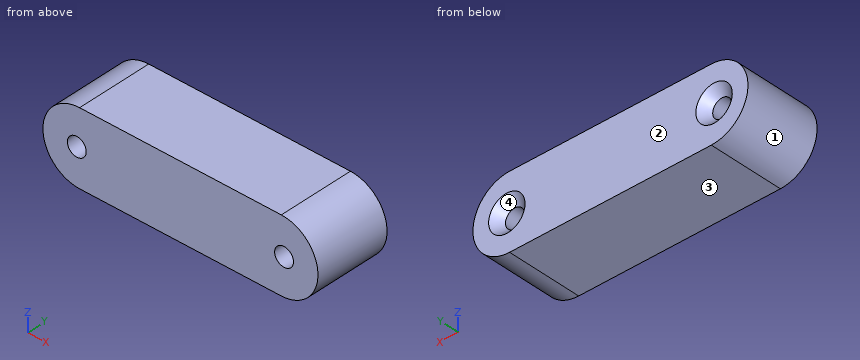
```python
from build123d import *

# Parameters (mm, degrees)
SKETCH1_R           = 1.905
BOSS_EXTRUDE1_DEPTH = 15.24
CHAMFER1_SIZE       = 1.778


with BuildPart() as part:
    # Sketch1 → Boss-Extrude1 (new body)
    with BuildSketch(Plane(origin=(0, 0, 0), x_dir=(1, 0, 0), z_dir=(0, 1, 0))):
        with BuildLine():
            Line((-20.3962, 7.4168), (20.3962, 7.4168))
            ThreePointArc((20.3962, 7.4168), (27.813, 0), (20.3962, -7.4168))
            Line((20.3962, -7.4168), (-20.3962, -7.4168))
            ThreePointArc((-20.3962, -7.4168), (-27.813, 0), (-20.3962, 7.4168))
        make_face()
        with Locations(Location((-20.955, 0, 0), (0, 0, 90))):
            Circle(SKETCH1_R, mode=Mode.SUBTRACT)
        with Locations(Location((20.955, 0, 0), (0, 0, 90))):
            Circle(SKETCH1_R, mode=Mode.SUBTRACT)
    extrude(amount=BOSS_EXTRUDE1_DEPTH)

    # Chamfer1
    chamfer1_edges = [part.edges().sort_by_distance(p)[0] for p in [
        (-20.955, 15.24, 1.905),
        (20.955, 15.24, 1.905),
    ]]
    chamfer(chamfer1_edges, length=CHAMFER1_SIZE)


solid = part.part
```
The model under review builds one solid part; all positions refer to its coordinate system, in mm. Face numbers are marked on the shaded views. Round coordinates to 2 decimals unless told otherwise and drop trailing zeros. Loops run counter-clockwise (first coordinate to the right, second up) from the corner with the lowest first, then second, coordinate; pieces in that order, holes last. Notation, with made-up numbers: (-24, 72.25) - (-17, 72.25) arc R19 cw to (-17, 96.25) - close; hole circle Ø3 at (-27, -35.75). An arc over 180 degrees is marked (long way). Use a Markdown table: item, result. Add a question column.
Q1. Add section A-A (z = 0). State the section outline as (x, y) points.
Q2. Add section C-C (z = -5.5). State the section outline as (x, y) points.
Q3. The part is to be moulded in two halves that separate along Z. For the marked faces 1, 2, 3 and 4, say which applies: pulls with the +Z half, pulls with the -Z half, needs draft (parallel to the pull), parting line crosses it, or undercut.
Q4. Insertion check: pin 1 Ø6 at (x, z) = (-20.955, 0) entering from +Y; pin 2 Ø3 at (y, z) = (11, 5) entering from +X; pin 3 Ø2 at (y, z) = (12.5, 5) entering from -X. Each pin has a flat end and moves straight along its axis. Give the tip position at first contact, or say it passes through.
Q5. For probe 1 along X at (y, z) = (8.25, 0); probe 2 along X at (y, z) = (3.75, -0.5); probe 3 along Z at (x, y) = (23, 14.5), list the stretches that pass through material, from the lowest coordinate up.
Q6. Add section B-B (y = 2). State the section outline as (x, z) points (3 decimals), plus the area to 3 significant figures.
Worked answers:
| question | item | result |
|---|---|---|
| 1 | outline | (-27.81, 0) - (-22.86, 0) - (-22.86, 13.46) - (-24.64, 15.24) - (-27.81, 15.24) - close; (-19.05, 0) - (19.05, 0) - (19.05, 13.46) - (17.27, 15.24) - (-17.27, 15.24) - (-19.05, 13.46) - close; (22.86, 0) - (27.81, 0) - (27.81, 15.24) - (24.64, 15.24) - (22.86, 13.46) - close |
| 2 | outline | (-25.37, 0) - (25.37, 0) - (25.37, 15.24) - (-25.37, 15.24) - close |
| 3 | face 1 | parting line crosses it |
| 3 | face 2 | needs draft |
| 3 | face 3 | pulls with the -Z half |
| 3 | face 4 | undercut |
| 4 | pin 1 | y = 14.56 |
| 4 | pin 2 | x = 26.94 |
| 4 | pin 3 | x = -26.64 |
| 5 | probe 1 | -27.81 to -22.86, -19.05 to 19.05, 22.86 to 27.81 |
| 5 | probe 2 | -27.8 to -22.79, -19.12 to 19.12, 22.79 to 27.8 |
| 5 | probe 3 | -6.94 to -2.12, 2.12 to 6.94 |
| 6 | outline | (-20.396, -7.417) - (20.396, -7.417) arc R7.417 ccw to (20.396, 7.417) - (-20.396, 7.417) arc R7.417 ccw to start; hole circle Ø3.81 at (-20.955, 0); hole circle Ø3.81 at (20.955, 0) |
| 6 | area | 755 mm² |
